from build123d import *

# Parameters (mm, degrees)
BOX310_W     = 3.4
BOX310_H     = 6.5
BOX310_DEPTH = 1.2
BOX309_W     = 3.4
BOX309_H     = 6.5
BOX309_DEPTH = 1.2
BOX308_W     = 4.4
BOX308_H     = 6.5
BOX308_DEPTH = 2.2


with BuildPart() as cubo295:
    # Box310 → Box310 (new body)
    with BuildSketch(Plane(origin=(15.8, -32, 13), x_dir=(0, 0, -1), z_dir=(1, 0, 0))):
        with Locations((1.7, 3.25)):
            Rectangle(BOX310_W, BOX310_H)
    extrude(amount=BOX310_DEPTH)


with BuildPart() as cubo294:
    # Box309 → Box309 (new body)
    with BuildSketch(Plane(origin=(14.7, -27, 10.26), x_dir=(1, 0, 0), z_dir=(0, 0, 1))):
        with Locations((1.7, 3.25)):
            Rectangle(BOX309_W, BOX309_H)
    extrude(amount=BOX309_DEPTH)


with BuildPart() as obj1:
    # Box308 → Box308 (new body)
    with BuildSketch(Plane(origin=(14.2, -26.9, 9.8), x_dir=(1, 0, 0), z_dir=(0, 0, 1))):
        with Locations((2.2, 3.25)):
            Rectangle(BOX308_W, BOX308_H)
    extrude(amount=BOX308_DEPTH)

    # Cut350: cut Cubo294
    add(cubo294.part, mode=Mode.SUBTRACT)

    # Cut351: cut Cubo295
    add(cubo295.part, mode=Mode.SUBTRACT)


with BuildPart() as obj1_1:
    # Cut351 placement: moved
    add(obj1.part.moved(Location((-2.4, 0, -2.4))))


solid = obj1_1.part
CAD build for the part. Positions are in the model's coordinates, mm. A direction names the side the tool comes from. Give positions to 0.01 mm unless a question says otherwise; leave off trailing zeros. Loops run counter-clockwise (first coordinate to the right, second up) from the corner with the lowest first, then second, coordinate; pieces in that order, holes last. Notation, with made-up numbers: M -25,29 L 10,29 A14 ccw 10,53 Z; hole C 63,75 d8. An arc over 180 degrees is marked long. Answer in a Markdown table with one row per item. Add a question column.
Item 1: Band-saw the part on D-D on y = -20.75. Give the cut face in (x, z), then the cut area to 3 significant figures.
Item 2: Band-saw the part on C-C on x = 15.25. Give the cut face in (y, z).
Item 3: Tool access for faces 5 (the face through (15.7, -23.7, 8.5)), 6 (the face through (14, -24, 9.6)): list every direction of +Z, -Z, +X, -X, +Y, -Y with a clear straight run to the whole face (end or side of a thin tool).
Item 4: Band-saw the part on B-B on z = 9.15. Give the cut face in (x, y), then the cut area to 3 significant figures.
Item 5: Band-saw the part on A-A on y = -26. Give the cut face in (x, z), then the cut area to 3 significant figures.
Item 6: Probe probe 1 along X at (y, z) = (-22.25, 9); probe 2 along Z at (x, y) = (14.2, -25); probe 3 along X at (y, z) = (-25.75, 9.3). List the from-to ranges inside material, lowest first.
Item 7: Mould opens along X. For faces 1 (the face through (12.3, -23.7, 8.5)), 2 (the face through (11.8, -24, 8)), 3 (the face through (16, -26.9, 8)), 4 (the face through (16.2, -24, 8)) say: +X half, -X half, draft (parallel to the pull), parting line (faces both ways), or undercut.
Item 8: Drop flat-ended pins along their axis: P1, Ø1, axis at x = 15, z = 9, coming from the -Y side; P2, Ø1, axis at x = 13.5, z = 8.5, coming from the -Y side. Give the stop position or say it passes through.
Reply:
| question | item | result |
|---|---|---|
| 1 | outline | M 11.8,7.4 L 16.2,7.4 L 16.2,9.6 L 11.8,9.6 Z; hole M 12.3,7.86 L 15.7,7.86 L 15.7,9.06 L 12.3,9.06 Z |
| 1 | area | 5.60 mm^2 |
| 2 | outline | M -26.9,7.4 L -20.4,7.4 L -20.4,9.6 L -26.9,9.6 L -26.9,9.06 L -20.5,9.06 L -20.5,7.86 L -26.9,7.86 Z |
| 3 | face 5 | -Y |
| 3 | face 6 | +Z, +X, -X, +Y, -Y |
| 4 | outline | M 11.8,-26.9 L 13.4,-26.9 L 13.4,-25.5 L 14.6,-25.5 L 14.6,-26.9 L 16.2,-26.9 L 16.2,-20.4 L 11.8,-20.4 Z |
| 4 | area | 26.9 mm^2 |
| 5 | outline | M 11.8,7.4 L 13.4,7.4 L 13.4,7.86 L 12.3,7.86 L 12.3,9.06 L 13.4,9.06 L 13.4,9.6 L 11.8,9.6 Z; M 14.6,7.4 L 16.2,7.4 L 16.2,9.6 L 14.6,9.6 L 14.6,9.06 L 15.7,9.06 L 15.7,7.86 L 14.6,7.86 Z |
| 5 | area | 4.40 mm^2 |
| 6 | probe 1 | x = 11.8 to 12.3, 15.7 to 16.2 |
| 6 | probe 2 | z = 7.4 to 7.86, 9.06 to 9.6 |
| 6 | probe 3 | x = 11.8 to 13.4, 14.6 to 16.2 |
| 7 | face 1 | undercut |
| 7 | face 2 | -X half |
| 7 | face 3 | draft |
| 7 | face 4 | +X half |
| 8 | P1 | stops at y = -26.9 |
| 8 | P2 | stops at y = -20.5 |
